from build123d import *


with BuildPart() as part:
    # Sketch1 → Revolve1 (revolve)
    with BuildSketch(Plane.XY):
        with BuildLine():
            Line((114.170121614, -21.739380235), (117.046248252, -11.00552949))
            Line((117.046248252, -11.00552949), (116.034199468, -10.734351836))
            Line((116.034199468, -10.734351836), (116.313594627, -9.691634906))
            Line((116.313594627, -9.691634906), (116.558939787, -9.757374944))
            Line((116.558939787, -9.757374944), (116.47676474, -10.064056394))
            ThreePointArc((116.47676474, -10.064056394), (116.527514155, -10.449536469), (116.835974985, -10.686226788))
            Line((116.835974985, -10.686226788), (116.86664313, -10.694444293))
            ThreePointArc((116.86664313, -10.694444293), (117.17510396, -10.931134613), (117.225853375, -11.316614688))
            Line((117.225853375, -11.316614688), (114.415466774, -21.805120272))
            Line((114.415466774, -21.805120272), (114.170121614, -21.739380235))
        make_face()
    revolve(axis=Axis((111.07814933, -7.762881267, 0), (-0.258819045, -0.965925826, 0)))


solid = part.part
CAD build for the part. Positions are in the model's coordinates, mm. Round coordinates to 2 decimals unless told otherwise and drop trailing zeros.
(1) Drop flat-ended pins along their axis: pin 1 (6 mm diameter, centred on x = 110, z = -2, fed in from +Y); pin 2 (8 mm diameter, centred on y = -10.5, z = 2, fed in from -X); pin 3 (2 mm diameter, centred on y = -16.5, z = 3.5, fed in from +X); pin 4 (1.5 mm diameter, centred on x = 113.5, y = -20, fed in from +Z). Give the stop position or say it passes through.
(2) Wall check: line 1 along Z through (x, y) = (109, -16.5); line 2 along Z through (x, y) = (106, -12.75); line 3 along X through (y, z) = (-13.25, -3). Give the ranges that are in metal, low to high.
(3) Two-plate mould, pull along Y, no slides. Class faces 1 (the cylindrical face through (116.1, -9.8, -2.2)), 2 (the cylindrical face through (105.447, -7.331, 0.244)): +Y half, -Y half, draft (parallel to the pull), parting line (faces both ways), or undercut.
Findings below:
1. pin 1: passes through
1. pin 2: stops at x = 102.27
1. pin 3: stops at x = 115.43
1. pin 4: stops at z = 4.94
2. line 1: z = -6.85 to -6.6, 6.6 to 6.85
2. line 2: z = -5.83 to -5.53, 5.53 to 5.83
2. line 3: x = 103.22 to 103.52, 115.7 to 115.99
3. face 1: undercut
3. face 2: parting line
